The drawing under review shows one solid part. Ordinate dimensions are in mm from its lowest x, y, z. Round coordinates to 2 decimals unless told otherwise and drop trailing zeros. Order: outer loops, then holes, each group sorted by start corner. A loop starts at its lowest first (then second) coordinate and runs counter-clockwise, first axis right, second up. Notation, with made-up numbers: (-6.5, -2.75) -> (9.5, -2.75) arc R19 cw to (9.5, 8.25) -> close; hole circle Ø6 at (-2.75, 61.25). An arc over 180 degrees is marked (long way). Use a Markdown table: item, result. Add a question column.
1) Wall thickness on line 1 along Y through (x, z) = (164, 19.5); line 2 along X through (y, z) = (5, 105.5); line 3 along X through (y, z) = (10.25, 99) (1 decimal): over which ranges is each line inside the solid? List them lowest first. Write a range as [from, to].
2) Consider section B-B (x = 107). State the section outline as (y, z) points.
3) Clearance check with flat-ended pins moving along their axes: P1, Ø3, axis at x = 231.5, y = 5, coming from the -Z side; P2, Ø10, axis at x = 155, z = 34, coming from the -Y side; P3, Ø3, axis at x = 227.5, y = 6.5, coming from the +Z side. State where each tip first meets the part, or that it passes through.
4) Consider section C-C (z = 72.5). State the section outline as (x, y) points, plus the area to 3 significant figures.
5) Consider section A-A (y = 3.25). State the section outline as (x, z) points.
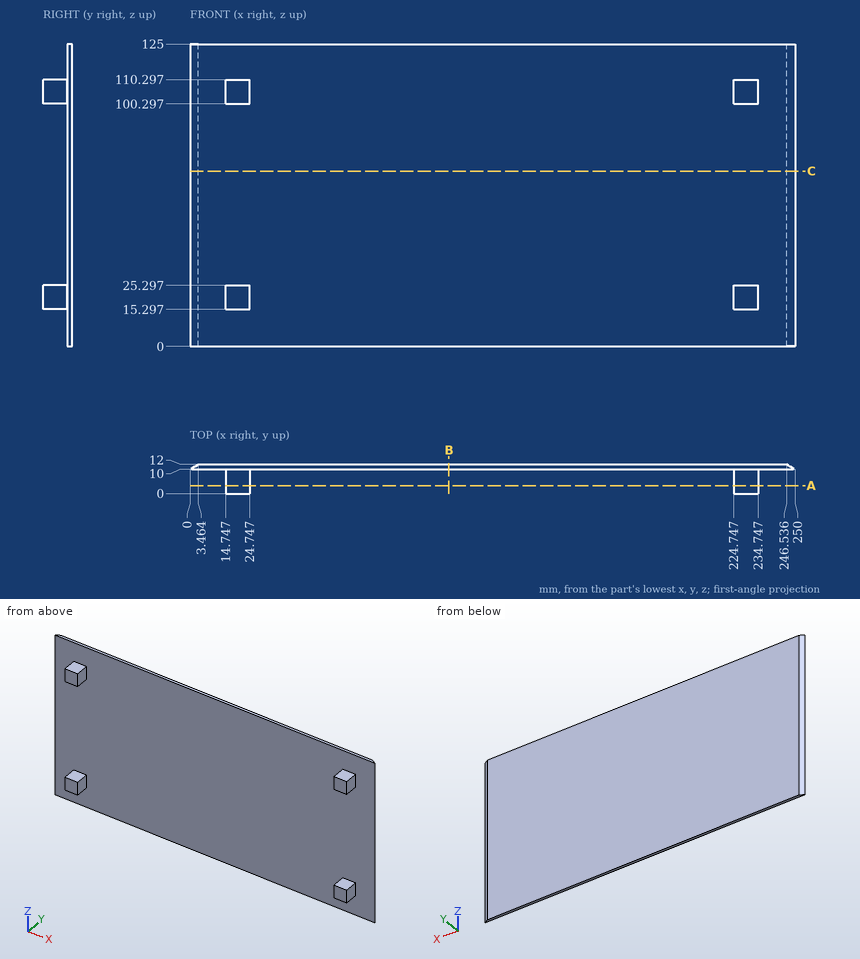
Results list:
| question | item | result |
|---|---|---|
| 1 | line 1 | [10, 12] |
| 1 | line 2 | [14.75, 24.75], [224.75, 234.75] |
| 1 | line 3 | [0.4, 249.6] |
| 2 | outline | (10, 0) -> (12, 0) -> (12, 125) -> (10, 125) -> close |
| 3 | P1 | z = 15.3 |
| 3 | P2 | y = 10 |
| 3 | P3 | z = 110.3 |
| 4 | outline | (0, 10) -> (250, 10) -> (246.54, 12) -> (3.46, 12) -> close |
| 4 | area | 493 mm2 |
| 5 | outline | (14.75, 15.3) -> (24.75, 15.3) -> (24.75, 25.3) -> (14.75, 25.3) -> close; (14.75, 100.3) -> (24.75, 100.3) -> (24.75, 110.3) -> (14.75, 110.3) -> close; (224.75, 15.3) -> (234.75, 15.3) -> (234.75, 25.3) -> (224.75, 25.3) -> close; (224.75, 100.3) -> (234.75, 100.3) -> (234.75, 110.3) -> (224.75, 110.3) -> close |
